from build123d import *

# Parameters (mm, degrees)
IZIM1_W                     = 75
IZIM1_H                     = 36
Y_KSEKLIK_EKSTR_ZYON1_DEPTH = 35
IZIM2_W                     = 50
IZIM2_H                     = 25
KES_EKSTR_ZYON1_DEPTH       = 36
IZIM6_R                     = 8
KES_EKSTR_ZYON3_DEPTH       = 5
KES_EKSTR_ZYON4_DEPTH       = 3
KES_EKSTR_ZYON5_DEPTH       = 26
KES_EKSTR_ZYON5_DEPTH_BACK  = 12
RADYUS2_R                   = 3
RADYUS3_R                   = 3
KES_EKSTR_ZYON7_DEPTH       = 36


with BuildPart() as part:
    # Çizim1 → Yükseklik-Ekstrüzyon1 (new body)
    with BuildSketch(Plane.XY):
        with Locations((37.5, 18)):
            Rectangle(IZIM1_W, IZIM1_H)
    extrude(amount=Y_KSEKLIK_EKSTR_ZYON1_DEPTH)

    # Çizim2 → Kes-Ekstrüzyon1 (cut, through all)
    with BuildSketch(Plane.XY.offset(35)):
        with Locations((25, 23.5)):
            Rectangle(IZIM2_W, IZIM2_H)
    extrude(amount=-KES_EKSTR_ZYON1_DEPTH, mode=Mode.SUBTRACT)

    # Çizim6 → Kes-Ekstrüzyon3 (cut)
    with BuildSketch(Plane.XY.offset(35)):
        with Locations((62.5, 20)):
            Circle(IZIM6_R)
    extrude(amount=-KES_EKSTR_ZYON3_DEPTH, mode=Mode.SUBTRACT)

    # Çizim7 → Kes-Ekstrüzyon4 (cut)
    with BuildSketch(Plane(origin=(0, 11, 0), x_dir=(1, 0, 0), z_dir=(0, 1, 0))):
        with BuildLine():
            Line((0, -7), (20, -7))
            ThreePointArc((20, -7), (30.5, -17.5), (20, -28))
            Line((20, -28), (0, -28))
            Line((0, -28), (0, -25))
            Line((0, -25), (20, -25))
            ThreePointArc((20, -25), (27.5, -17.5), (20, -10))
            Line((20, -10), (0, -10))
            Line((0, -10), (0, -7))
        make_face()
    extrude(amount=-KES_EKSTR_ZYON4_DEPTH, mode=Mode.SUBTRACT)

    # Çizim8 → Kes-Ekstrüzyon5 (cut, two sides)
    with BuildSketch(Plane(origin=(0, 11, 0), x_dir=(1, 0, 0), z_dir=(0, 1, 0))) as kes_ekstr_zyon5_sk:
        with BuildLine():
            Line((0, -10), (20, -10))
            ThreePointArc((20, -10), (27.5, -17.5), (20, -25))
            Line((20, -25), (0, -25))
            Line((0, -25), (0, -10))
        make_face()
    extrude(amount=KES_EKSTR_ZYON5_DEPTH, mode=Mode.SUBTRACT)
    extrude(kes_ekstr_zyon5_sk.sketch, amount=-KES_EKSTR_ZYON5_DEPTH_BACK, mode=Mode.SUBTRACT)

    # Radyus2
    radyus2_edges = [part.edges().sort_by_distance(p)[0] for p in [
        (0, 5.5, 0),
    ]]
    fillet(radyus2_edges, radius=RADYUS2_R)

    # Radyus3
    radyus3_edges = [part.edges().sort_by_distance(p)[0] for p in [
        (0, 5.5, 35),
    ]]
    fillet(radyus3_edges, radius=RADYUS3_R)

    # Çizim9 → Kes-Ekstrüzyon7 (cut, through all)
    with BuildSketch(Plane.XY.offset(35)):
        with BuildLine():
            Line((50, 20), (50, 36))
            Line((50, 36), (75, 36))
            Line((75, 36), (75, 20))
            ThreePointArc((75, 20), (62.5, 32.5), (50, 20))
        make_face()
    extrude(amount=-KES_EKSTR_ZYON7_DEPTH, mode=Mode.SUBTRACT)


solid = part.part
Check sheet for the modelled part. Datum: model origin and axes. Units: mm. A direction names the side the tool comes from. Give positions to 0.01 mm unless a question says otherwise; leave off trailing zeros. Write each loop counter-clockwise with the first axis right and the second up, starting at its lowest first coordinate (ties: lowest second). Pieces come first, ordered by that corner, then holes. Notation, with made-up numbers: (-37, -1.5) -> (-15, -1.5) arc R28 cw to (-15, 32.5) -> close; hole circle Ø4 at (56.25, 54). An arc over 180 degrees is marked (long way). One line per item, written item: value. Start each with the question number.
Item 1: Section check C-C on y = 5. Record the cut outline in (x, z).
Item 2: Draft check along X on faces 1 (the cylindrical face through (54.508, 20.352, 32.535)), 2 (the flat face through (75, 10, 17)), 3 (the flat face through (50, 15, 18)), 4 (the flat face through (37, 0, 17)). Enter one of: +X half, -X half, draft (parallel to the pull), parting line (faces both ways), or undercut.
Item 3: Gauge pin test, flat ends, axial feed: pin 1 (8 mm diameter, centred on x = 38.5, z = 12.5, fed in from +Y); pin 2 (3 mm diameter, centred on x = 66.5, z = 3.5, fed in from -Y); pin 3 (1.5 mm diameter, centred on x = 10, z = 24, fed in from -Y); pin 4 (17 mm diameter, centred on x = 16, z = 17, fed in from +Y). Record the tip position at first contact, or that the pin passes through.
Item 4: Section check A-A on x = 10. Record the cut outline in (y, z), then the cut area to 3 significant figures.
Item 5: Section check B-B on x = 62.5. Record the cut outline in (y, z).
Item 6: Section check D-D on z = 6. Record the cut outline in (x, y), then the cut area to 3 significant figures.
Item 7: Material ranges on probe 1 along Z at (x, y) = (16, 7); probe 2 along Y at (x, z) = (62.5, 31.75); probe 3 along Y at (x, z) = (40.5, 9), recorded low to high. Write a range as from..to.
Item 8: Tool access check on faces 5 (the flat face through (30.2, 11, 13.9)), 6 (the flat face through (10, 4, 10)), 7 (the flat face through (62, 20, 30)), 8 (the flat face through (10, 10, 28)). Record the directions out of +Z, -Z, +X, -X, +Y, -Y that give a thin tool (end or side, any length) a straight path to the whole face; none if there is none.
Results list:
1. outline: (0, 3) arc R3 ccw to (3, 0) -> (75, 0) -> (75, 35) -> (3, 35) arc R3 ccw to (0, 32) -> (0, 25) -> (20, 25) arc R7.5 cw to (20, 10) -> (0, 10) -> close
2. face 1: undercut
2. face 2: +X half
2. face 3: -X half
2. face 4: draft
3. pin 1: y = 11
3. pin 2: y = 0
3. pin 3: through
3. pin 4: y = 8
4. outline: (0, 0) -> (11, 0) -> (11, 7) -> (8, 7) -> (8, 10) -> (0, 10) -> close; (0, 25) -> (8, 25) -> (8, 28) -> (11, 28) -> (11, 35) -> (0, 35) -> close
4. area: 202 mm²
5. outline: (0, 0) -> (32.5, 0) -> (32.5, 35) -> (28, 35) -> (28, 30) -> (12, 30) -> (12, 35) -> (0, 35) -> close
6. outline: (0, 0) -> (75, 0) -> (75, 20) arc R12.5 ccw to (50, 20) -> (50, 11) -> (0, 11) -> close
6. area: 1,300 mm²
7. probe 1: 0..10, 25..35
7. probe 2: 0..12, 28..32.5
7. probe 3: 0..11
8. face 5: +Z, -Z, -X, +Y
8. face 6: -X, +Y, -Y
8. face 7: +Z
8. face 8: -X, +Y
